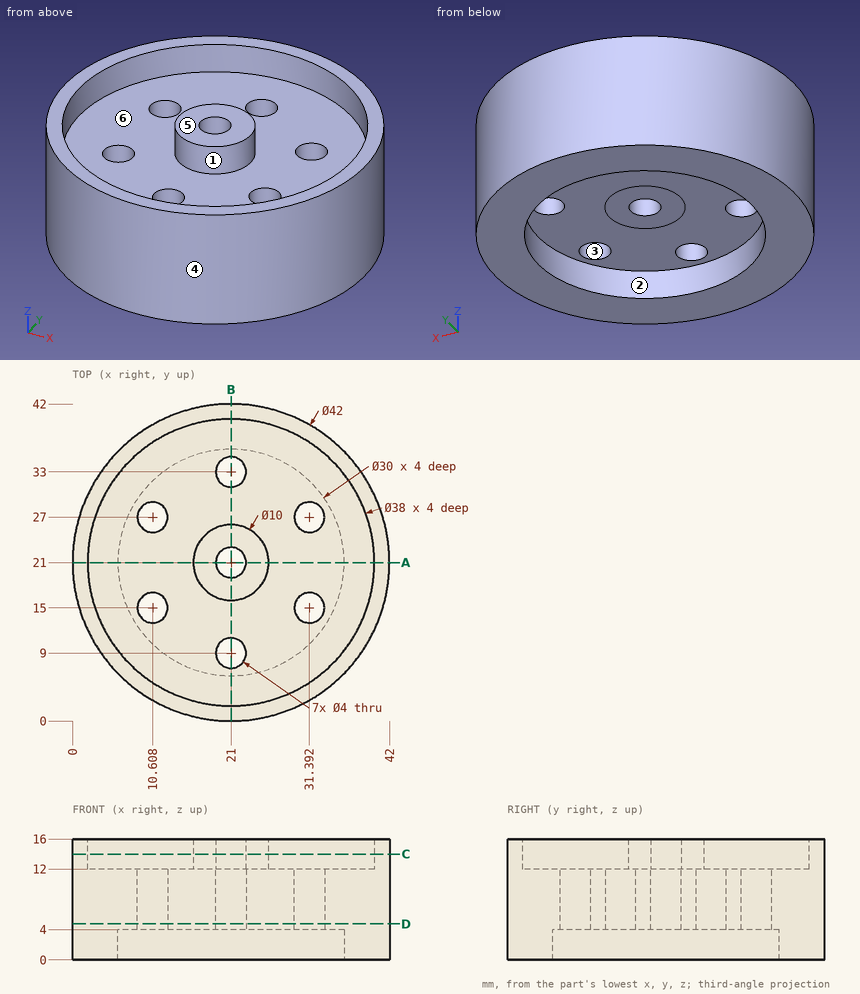
Verification items for this drawing (mm, ordinates from the low corner). A direction names the side the tool comes from. Coordinates: 2 decimals unless noted, no trailing zeros. Order: outer loops, then holes, each group sorted by start corner. A loop starts at its lowest first (then second) coordinate and runs counter-clockwise, first axis right, second up. Notation, with made-up numbers: (56, 28.25) - (115, 28.25) arc R16 ccw to (115, 55.25) - close; hole circle Ø3 at (-31, 28). An arc over 180 degrees is marked (long way). Answer in a Markdown table with one row per item. Add a question column.
1. Gauge pin test, flat ends, axial feed: pin 1 Ø5 at (x, z) = (30.5, 14) entering from -Y; pin 2 Ø4 at (x, z) = (18, 12.5) entering from -Y; pin 3 Ø23 at (x, y) = (21, 21) entering from -Z. Record the tip position at first contact, or that the pin passes through.
2. Access from +Z, -Z, +X, -X, +Y, -Y to the whole of each face (thin tool, end or side, straight path). Record for the marked faces 1, 2 and 3.
3. Draft check along X on the marked faces 4, 5 and 6. Enter one of: +X half, -X half, draft (parallel to the pull), parting line (faces both ways), or undercut.
4. Section check D-D (z = 4.75). Enter the section's corners in (x, y), plus the area to 3 significant figures.
5. Section check B-B (x = 21). Enter the section's corners in (y, z).
6. Section check C-C (z = 14). Enter the section's corners in (x, y).
7. Section check A-A (y = 21). Enter the section's corners in (x, z).
8. Material ranges on L1, parallel to Y at x = 21, z = 6; L2, parallel to X at y = 28, z = 10.5 (1 decimal); L3, parallel to Z at x = 22, y = 4.5, recorded low to high. Write a range as [from, to].
Data:
| question | item | result |
|---|---|---|
| 1 | pin 1 | stops at y = 1.2 |
| 1 | pin 2 | stops at y = 0.02 |
| 1 | pin 3 | stops at z = 4 |
| 2 | face 1 | +Z |
| 2 | face 2 | -Z |
| 2 | face 3 | +Z, -Z |
| 3 | face 4 | parting line |
| 3 | face 5 | draft |
| 3 | face 6 | undercut |
| 4 | outline | circle Ø42 at (21, 21); hole circle Ø4 at (10.61, 15); hole circle Ø4 at (10.61, 27); hole circle Ø4 at (21, 9); hole circle Ø4 at (21, 21); hole circle Ø4 at (21, 33); hole circle Ø4 at (31.39, 15); hole circle Ø4 at (31.39, 27) |
| 4 | area | 1,300 mm² |
| 5 | outline | (0, 0) - (6, 0) - (6, 4) - (7, 4) - (7, 12) - (2, 12) - (2, 16) - (0, 16) - close; (11, 4) - (19, 4) - (19, 16) - (16, 16) - (16, 12) - (11, 12) - close; (23, 4) - (31, 4) - (31, 12) - (26, 12) - (26, 16) - (23, 16) - close; (35, 4) - (36, 4) - (36, 0) - (42, 0) - (42, 16) - (40, 16) - (40, 12) - (35, 12) - close |
| 6 | outline | circle Ø42 at (21, 21); circle Ø10 at (21, 21); hole circle Ø38 at (21, 21); hole circle Ø4 at (21, 21) |
| 7 | outline | (0, 0) - (6, 0) - (6, 4) - (19, 4) - (19, 16) - (16, 16) - (16, 12) - (2, 12) - (2, 16) - (0, 16) - close; (23, 4) - (36, 4) - (36, 0) - (42, 0) - (42, 16) - (40, 16) - (40, 12) - (26, 12) - (26, 16) - (23, 16) - close |
| 8 | L1 | y = [0, 7], [11, 19], [23, 31], [35, 42] |
| 8 | L2 | x = [1.2, 8.9], [12.3, 29.7], [33.1, 40.8] |
| 8 | L3 | z = [0, 12] |
